Autodesk Inventor part; units mm, degrees
ref_plane "YZ Plane" through (0, 0, 0) normal (1, 0, 0) x (0, 1, 0)
ref_plane "XZ Plane" through (0, 0, 0) normal (0, 1, 0) x (-1, 0, 0)
ref_plane "XY Plane" through (0, 0, 0) normal (0, 0, 1) x (1, 0, 0)
sketch "Sketch6" plane through (0, 0, 0) normal (0, 0, 1) x (1, 0, 0)
  line L0 (11.35, 0) -> (11.35, 1.7)
  line L1 (11.35, 1.7) -> (11.6, 1.7)
  line L2 (11.6, 1.7) -> (11.6, 20.5)
  line L3 (11.6, 20.5) -> (12.5, 20.5)
  line L4 (12.5, 20.5) -> (12.5, 33.9)
  line L5 (12.5, 33.9) -> (13.25, 33.9)
  line L6 (13.25, 33.9) -> (13.25, 36.2)
  line L7 (11.35, 0) -> (9.75, 0)
  line L8 (9.75, 0) -> (9.75, 33.9)
  line L9 (13.25, 36.2) -> (5.15, 36.2)
  line L10 (5.15, 36.2) -> (5.15, 33.9)
  line L11 (5.15, 33.9) -> (9.75, 33.9)
  line L12 (0, -7.24) -> (0, 43.44) construction
  point P0 (0, 0)
  dimension "d7" = 11.35
  dimension "d8" = 1.7
  dimension "d9" = 11.6
  dimension "d11" = 12.5
  dimension "d13" = 13.25
  dimension "d14" = 2.3
  dimension "d16" = 1.6
  dimension "d17" = 8.1
  dimension "d18" = 0.25
  dimension "d19" = 15.7
  dimension "d20" = 36.2
revolve "Revolution1" add sketch "Sketch6" angle 360 about axis through (0, -10, 0) along (0, 1, 0)
properties part number "Eye-Piece"
Geometry: final body of the model. Coordinates: model frame, mm. A direction names the side the tool comes from. Round coordinates to 2 decimals unless told otherwise and drop trailing zeros. Loops run counter-clockwise (first coordinate to the right, second up) from the corner with the lowest first, then second, coordinate; pieces in that order, holes last. Notation, with made-up numbers: M -29,84 L -1,84 A18 cw -1,106 Z; hole C 44,61.25 d2. An arc over 180 degrees is marked long. Put each result on its own line as item: value. Start each with the question number.
(1) Set-up query: faces 4 (the face through (11.923, 27.294, -3.755)), 5 (the face through (6, 36.2, 0)). Return all of +Z, -Z, +X, -X, +Y, -Y with unobstructed straight access to the full face (end or side cutting, diameter ignored); none if empty.
(2) Draft query along Z for faces 1 (the face through (10, 33.9, -8)), 2 (the face through (10.485, 0.862, 4.347)), 3 (the face through (-1.269, 17.187, -9.667)). Return one class per face: +Z half, -Z half, draft (parallel to the pull), parting line (faces both ways), or undercut.
(3) Section query B-B (x = 0). Return loops of the section in (y, z).
(4) Contact query for flat-ended pins moving along their axis: pin 1 Ø1.5 at (x, y) = (-7.5, 28) entering from +Z; pin 2 Ø5 at (x, y) = (4.5, 18.5) entering from +Z; pin 3 Ø8 at (y, z) = (9.5, -6.5) entering from +X. Output: stop coordinate, or through.
(5) Section query C-C (y = 23). Return loops of the section in (x, z).
(6) Section query D-D (z = -10.75). Return loops of the section in (x, y).
(7) Section query A-A (z = 0). Return loops of the section in (x, y), then the cut area to 3 significant figures.
(8) Material intervals for line 1 along Z through (x, y) = (0, 35.15); line 2 along Z through (x, y) = (0.25, 32.5); line 3 along X through (y, z) = (10, 0), sorted ascending. Write a range as [from, to].
Findings below:
1. face 4: -Y
1. face 5: +Z, -Z, +X, -X, +Y
2. face 1: draft
2. face 2: parting line
2. face 3: undercut
3. outline: M 0,-11.35 L 1.7,-11.35 L 1.7,-11.6 L 20.5,-11.6 L 20.5,-12.5 L 33.9,-12.5 L 33.9,-13.25 L 36.2,-13.25 L 36.2,-5.15 L 33.9,-5.15 L 33.9,-9.75 L 0,-9.75 Z; M 0,9.75 L 33.9,9.75 L 33.9,5.15 L 36.2,5.15 L 36.2,13.25 L 33.9,13.25 L 33.9,12.5 L 20.5,12.5 L 20.5,11.6 L 1.7,11.6 L 1.7,11.35 L 0,11.35 Z
4. pin 1: stops at z = 10.52
4. pin 2: stops at z = 12.13
4. pin 3: stops at x = 11.33
5. outline: C 0,0 d25; hole C 0,0 d19.5
6. outline: M -7.75,33.9 L -6.38,33.9 L -6.38,20.5 L -4.36,20.5 L -4.36,1.7 L -3.64,1.7 L -3.64,0 L 3.64,0 L 3.64,1.7 L 4.36,1.7 L 4.36,20.5 L 6.38,20.5 L 6.38,33.9 L 7.75,33.9 L 7.75,36.2 L -7.75,36.2 Z
7. outline: M -13.25,33.9 L -12.5,33.9 L -12.5,20.5 L -11.6,20.5 L -11.6,1.7 L -11.35,1.7 L -11.35,0 L -9.75,0 L -9.75,33.9 L -5.15,33.9 L -5.15,36.2 L -13.25,36.2 Z; M 5.15,33.9 L 9.75,33.9 L 9.75,0 L 11.35,0 L 11.35,1.7 L 11.6,1.7 L 11.6,20.5 L 12.5,20.5 L 12.5,33.9 L 13.25,33.9 L 13.25,36.2 L 5.15,36.2 Z
7. area: 186 mm2
8. line 1: z = [-13.25, -5.15], [5.15, 13.25]
8. line 2: z = [-12.5, -9.75], [9.75, 12.5]
8. line 3: x = [-11.6, -9.75], [9.75, 11.6]
